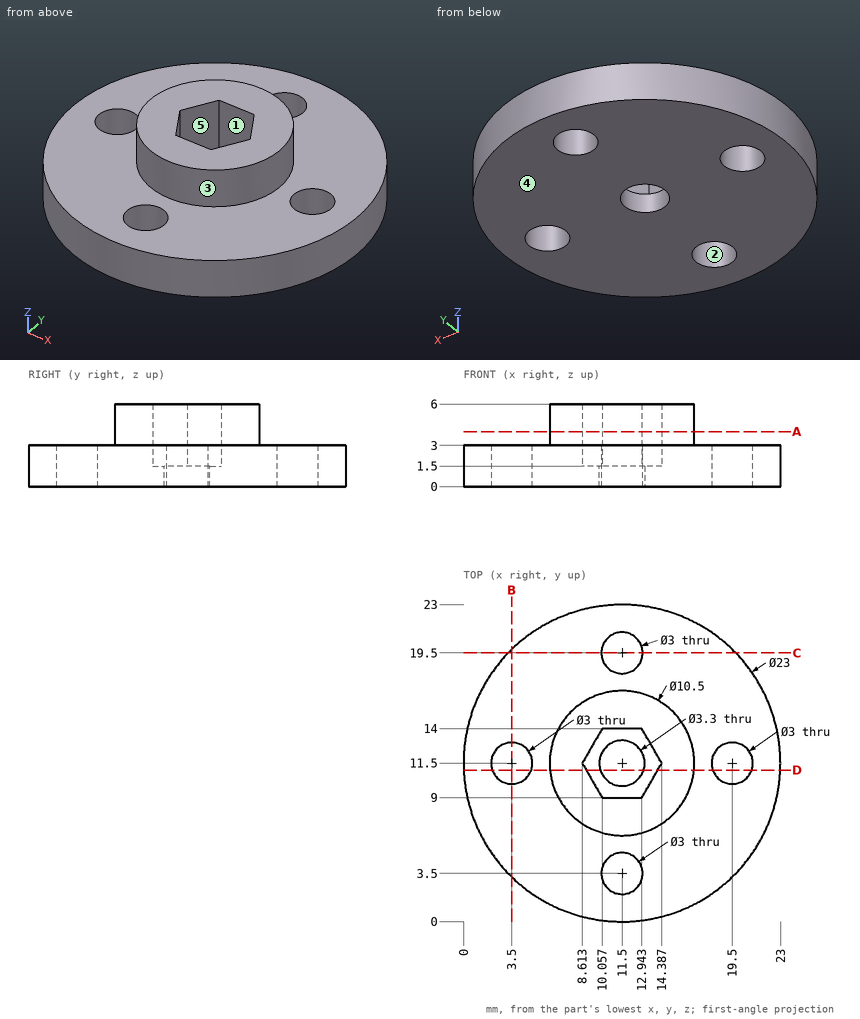
The drawing under review shows one solid part. Ordinate dimensions are in mm from its lowest x, y, z. A direction names the side the tool comes from. Round coordinates to 2 decimals unless told otherwise and drop trailing zeros. Write each loop counter-clockwise with the first axis right and the second up, starting at its lowest first coordinate (ties: lowest second). Pieces come first, ordered by that corner, then holes. Notation, with made-up numbers: (-27, -0.5) - (7, -0.5) arc R14 cw to (7, 8.5) - close; hole circle Ø9 at (-32.5, 63). An arc over 180 degrees is marked (long way). Use a Markdown table: item, result. Add a question column.
1. We need section A-A (z = 4). State the section outline as (x, y) points.
2. Wall thickness on probe 1 along Y at (x, z) = (11.5, 2.9); probe 2 along Y at (x, z) = (8.75, 5.55) (1 decimal); probe 3 along Z at (x, y) = (15.5, 17.5): over which ranges is each line inside the solid? List them lowest first.
3. Clearance check with flat-ended pins moving along their axes: pin 1 (10 mm diameter, centred on x = 20.5, y = 18.5, fed in from -Z); pin 2 (4.5 mm diameter, centred on x = 11.5, y = 11.5, fed in from +Z); pin 3 (1.5 mm diameter, centred on y = 5.5, z = 2, fed in from +X); pin 4 (1 mm diameter, centred on y = 8.5, z = 3, fed in from +X) (1 decimal). State where each tip first meets the part, or that it passes through.
4. We need section B-B (x = 3.5). State the section outline as (y, z) points.
5. We need section D-D (y = 11). State the section outline as (x, z) points.
6. Mouldability with a two-part tool opening along X and no side actions: class the marked faces 3, 4 and 5 as +X half, -X half, draft (parallel to the pull), parting line (faces both ways), or undercut.
7. For the marked faces 1 and 2, list the 3-axis set-ups (+Z, -Z, +X, -X, +Y, -Y) from which the entire face can be reached by the end or side of a thin tool; tool diameter is ignored.
Output:
| question | item | result |
|---|---|---|
| 1 | outline | circle Ø10.5 at (11.5, 11.5); hole (8.61, 11.5) - (10.06, 9) - (12.94, 9) - (14.39, 11.5) - (12.94, 14) - (10.06, 14) - close |
| 2 | probe 1 | y = 0 to 2, 5 to 9, 14 to 18, 21 to 23 |
| 2 | probe 2 | y = 7 to 11.3, 11.7 to 16 |
| 2 | probe 3 | z = 0 to 3 |
| 3 | pin 1 | stops at z = 0 |
| 3 | pin 2 | stops at z = 1.5 |
| 3 | pin 3 | stops at x = 21.73 |
| 3 | pin 4 | stops at x = 22.7 |
| 4 | outline | (3.24, 0) - (10, 0) - (10, 3) - (3.24, 3) - close; (13, 0) - (19.76, 0) - (19.76, 3) - (13, 3) - close |
| 5 | outline | (0.01, 0) - (2.09, 0) - (2.09, 3) - (0.01, 3) - close; (4.91, 0) - (9.93, 0) - (9.93, 1.5) - (8.9, 1.5) - (8.9, 6) - (6.27, 6) - (6.27, 3) - (4.91, 3) - close; (13.07, 0) - (18.09, 0) - (18.09, 3) - (16.73, 3) - (16.73, 6) - (14.1, 6) - (14.1, 1.5) - (13.07, 1.5) - close; (20.91, 0) - (22.99, 0) - (22.99, 3) - (20.91, 3) - close |
| 6 | face 3 | parting line |
| 6 | face 4 | draft |
| 6 | face 5 | undercut |
| 7 | face 1 | +Z |
| 7 | face 2 | +Z, -Z |
